Read the model definition and answer for the solid it produces. Units are mm, in the model's axes. Give positions to 0.01 mm unless a question says otherwise; leave off trailing zeros. Order: outer loops, then holes, each group sorted by start corner. A loop starts at its lowest first (then second) coordinate and runs counter-clockwise, first axis right, second up. Notation, with made-up numbers: (-1.75, 61) - (53.25, 61) arc R14 ccw to (53.25, 67) - close; hole circle Ø6 at (57.5, 10.25). An arc over 180 degrees is marked (long way). Write item = value, one per line.
```python
from build123d import *

# Parameters (mm, degrees)
SKETCH1_W           = 635.3556
SKETCH1_H           = 184.15
BOSS_EXTRUDE1_DEPTH = 1.5875
SKETCH2_W           = 210.6549
SKETCH2_H           = 3.175
BOSS_EXTRUDE2_DEPTH = 3.175
BOSS_EXTRUDE3_DEPTH = 3.175
CUT_EXTRUDE1_DEPTH  = 10
LPATTERN1_COUNT     = 5
LPATTERN1_PITCH     = 140.97


with BuildPart() as part:
    # Sketch1 → Boss-Extrude1 (new, symmetric)
    with BuildSketch(Plane(origin=(0, 0, 0), x_dir=(1, 0, 0), z_dir=(0, 1, 0))):
        Rectangle(SKETCH1_W, SKETCH1_H)
    extrude(amount=BOSS_EXTRUDE1_DEPTH, both=True)

    # Sketch2 → Boss-Extrude2 (add)
    with BuildSketch(Plane(origin=(0, 0, -92.075), x_dir=(-1, 0, 0), z_dir=(0, 0, -1))):
        with Locations((-136.15035, 0)):
            Rectangle(SKETCH2_W, SKETCH2_H)
        with Locations((136.15035, 0)):
            Rectangle(SKETCH2_W, SKETCH2_H)
    extrude(amount=BOSS_EXTRUDE2_DEPTH)

    # Sketch3 → Boss-Extrude3 (add)
    with BuildSketch(Plane(origin=(0, 1.5875, 0), x_dir=(1, 0, 0), z_dir=(0, 1, 0))):
        Polygon((-317.6778, 47.625), (-317.6778, 92.075), (-349.4278, 92.075), (-349.4278, 87.3125), align=None)
    boss_extrude3 = extrude(amount=-BOSS_EXTRUDE3_DEPTH)

    # Mirror1: Boss-Extrude3 across plane
    add(boss_extrude3.mirror(Plane(origin=(0, 0, 0), x_dir=(0, 0, 1), z_dir=(1, 0, 0))))

    # Sketch4 → Cut-Extrude1 (cut)
    with BuildSketch(Plane(origin=(0, 1.5875, 0), x_dir=(1, 0, 0), z_dir=(0, 1, 0))):
        with BuildLine():
            ThreePointArc((-275.2528, -81.534), (-274.659691232, -82.965891232), (-273.2278, -83.559))
            Line((-273.2278, -83.559), (-273.2278, -81.534))
            Line((-273.2278, -81.534), (-275.2528, -81.534))
        make_face()
        with BuildLine():
            Line((-273.2278, -81.534), (-273.2278, -83.559))
            ThreePointArc((-273.2278, -83.559), (-271.795908768, -82.965891232), (-271.2028, -81.534))
            ThreePointArc((-271.2028, -81.534), (-273.2278, -79.509), (-275.2528, -81.534))
            Line((-275.2528, -81.534), (-273.2278, -81.534))
        make_face()
    cut_extrude1 = extrude(amount=-CUT_EXTRUDE1_DEPTH, mode=Mode.SUBTRACT)

    # LPattern1: Cut-Extrude1 ×5
    with Locations(*[(i * LPATTERN1_PITCH, 0, 0) for i in range(1, LPATTERN1_COUNT)]):
        add(cut_extrude1, mode=Mode.SUBTRACT)


solid = part.part
```
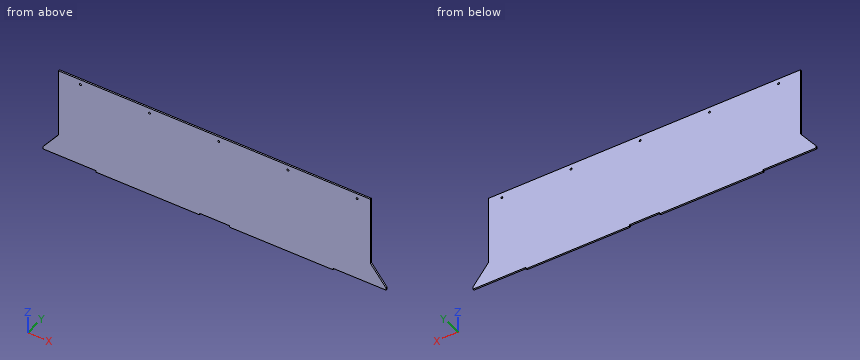
1. Section C-C (x = -299.5) is taken. Determine the outline of the cut face in (y, z) (1 decimal), and give its area (3 significant figures).
Recorded:
outline = (-1.6, -92.1) - (1.6, -92.1) - (1.6, 92.1) - (-1.6, 92.1) - close
area = 585 mm^2
2. Straight lines are drawn through the part: L1, parallel to X at y = -1.1, z = 2; L2, parallel to Z at x = -314.5, y = 1.35 (3 decimals); L3, parallel to X at y = -0.7, z = -86. For each, find the intervals that lie inside material, in ascending order. Write a range as [from, to].
Recorded:
L1 = [-317.68, 317.68]
L2 = [-92.075, 92.075]
L3 = [-348.38, 348.38]
3. Section A-A (y = -0.35) is taken. Count the separate pieces of the cut face and the enclosed holes in it, and give its area (3 significant figures).
Recorded:
separate_pieces = 1
enclosed_holes = 5
area = 120,000 mm^2
4. Section B-B (z = -26.5) is taken. Determine the outline of the cut face in (x, y).
Recorded:
outline = (-317.68, -1.59) - (317.68, -1.59) - (317.68, 1.59) - (-317.68, 1.59) - close
5. Flat-ended cylindrical pins translate along their axes: pin 1 (1 mm diameter, centred on y = 0, z = 36, fed in from +X); pin 2 (1.6 mm diameter, centred on x = -14, y = -0.5, fed in from -Z) (3 decimals). Find the tip coordinate at first contact, or state that the pin passes through.
Recorded:
pin_1 = 317.68
pin_2 = -92.075
